The listing builds one solid part. Answer for the finished solid, in the listing's coordinates (mm). Face numbers are marked on the shaded views. Coordinates: 2 decimals unless noted, no trailing zeros. Order: outer loops, then holes, each group sorted by start corner. A loop starts at its lowest first (then second) coordinate and runs counter-clockwise, first axis right, second up. Notation, with made-up numbers: (63, 53.25) -> (116, 53.25) arc R27 ccw to (116, 91.25) -> close; hole circle Ø4 at (53, 67). An arc over 180 degrees is marked (long way). Answer in a Markdown table with one row per item. Add a question column.
```python
from build123d import *

# Parameters (mm, degrees)
SKETCH1_W           = 321.435935394
SKETCH1_H           = 221.435935394
BOSS_EXTRUDE1_DEPTH = 30
FILLET1_R           = 20
SHELL1_T            = -2
CUT_EXTRUDE1_REACH  = 1355.856
SKETCH2_W           = 156.2
SKETCH2_H           = 88.6
SKETCH5_R           = 5
SKETCH5_R_2         = 1.5
BOSS_EXTRUDE2_DEPTH = 20
FILLET2_R           = 5


with BuildPart() as part:
    # Sketch1 → Boss-Extrude1 (new body)
    with BuildSketch(Plane(origin=(0, -69.673086457, -260.023498579), x_dir=(1, 0, 0), z_dir=(0, 0.2588190451025214, 0.9659258262890682))):
        with Locations((1020.211286357, 547.548055232)):
            Rectangle(SKETCH1_W, SKETCH1_H)
    extrude(amount=BOSS_EXTRUDE1_DEPTH)

    # Fillet1
    fillet1_edges = [part.edges().sort_by_distance(p)[0] for p in [
        (859.49331866, 466.982292579, -372.761588593),
        (1020.211286357, 360.036948146, -344.105669918),
        (1180.929254054, 466.982292579, -372.761588593),
        (1020.211286357, 573.927637012, -401.417507268),
    ]]
    fillet(fillet1_edges, radius=FILLET1_R)

    # Shell1
    shell1_openings = [part.faces().sort_by_distance(p)[0] for p in [
        (1020.211286357, 459.217721226, -401.739363381),
    ]]
    offset(amount=SHELL1_T, openings=shell1_openings)

    # Sketch2 → Cut-Extrude1 (cut, up to next)
    with BuildSketch(Plane(origin=(0, -61.908515104, -231.04572379), x_dir=(1, 0, 0), z_dir=(0, 0.2588190451025213, 0.9659258262890681)), mode=Mode.PRIVATE) as cut_extrude1_sk1:
        with Locations((1020.211286357, 547.548055232)):
            Rectangle(SKETCH2_W, SKETCH2_H)
    cut_extrude1_tool1 = extrude(cut_extrude1_sk1.sketch, amount=-CUT_EXTRUDE1_REACH, mode=Mode.PRIVATE) & part.part
    add(cut_extrude1_tool1.solids().sort_by_distance((1020.211286, 466.982293, -372.761589))[0], mode=Mode.SUBTRACT)

    # Sketch5 → Boss-Extrude2 (add)
    # profile 1 of 4: a face of its own
    with BuildSketch(Plane(origin=(0, -62.426153194, -232.977575442), x_dir=(-1, 0, 0), z_dir=(0, -0.25881904510252146, -0.9659258262890681))):
        with Locations(Location((-901.394461057, 616.364880532, 0), (0, 0, 270))):
            Circle(SKETCH5_R)
        with Locations(Location((-901.394461057, 616.364880532, 0), (0, 0, 90))):
            Circle(SKETCH5_R_2, mode=Mode.SUBTRACT)
    # profile 2 of 4: a face of its own
    with BuildSketch(Plane(origin=(0, -62.426153194, -232.977575442), x_dir=(-1, 0, 0), z_dir=(0, -0.25881904510252146, -0.9659258262890681))):
        with Locations(Location((-901.394461057, 478.731229931, 0), (0, 0, 270))):
            Circle(SKETCH5_R)
        with Locations(Location((-901.394461057, 478.731229931, 0), (0, 0, 90))):
            Circle(SKETCH5_R_2, mode=Mode.SUBTRACT)
    # profile 3 of 4: a face of its own
    with BuildSketch(Plane(origin=(0, -62.426153194, -232.977575442), x_dir=(-1, 0, 0), z_dir=(0, -0.25881904510252146, -0.9659258262890681))):
        with Locations(Location((-1139.028111658, 478.731229931, 0), (0, 0, 270))):
            Circle(SKETCH5_R)
        with Locations(Location((-1139.028111658, 478.731229931, 0), (0, 0, 90))):
            Circle(SKETCH5_R_2, mode=Mode.SUBTRACT)
    # profile 4 of 4: a face of its own
    with BuildSketch(Plane(origin=(0, -62.426153194, -232.977575442), x_dir=(-1, 0, 0), z_dir=(0, -0.25881904510252146, -0.9659258262890681))):
        with Locations(Location((-1139.028111658, 616.364880532, 0), (0, 0, 270))):
            Circle(SKETCH5_R)
        with Locations(Location((-1139.028111658, 616.364880532, 0), (0, 0, 90))):
            Circle(SKETCH5_R_2, mode=Mode.SUBTRACT)
    extrude(amount=BOSS_EXTRUDE2_DEPTH)

    # Fillet2
    fillet2_edges = [part.edges().sort_by_distance(p)[0] for p in [
        (901.394461057, 537.766232461, -393.798640482),
        (901.394461057, 404.822334779, -358.17643046),
        (1139.028111658, 404.822334779, -358.17643046),
        (1139.028111658, 537.766232461, -393.798640482),
    ]]
    fillet(fillet2_edges, radius=FILLET2_R)


solid = part.part
```
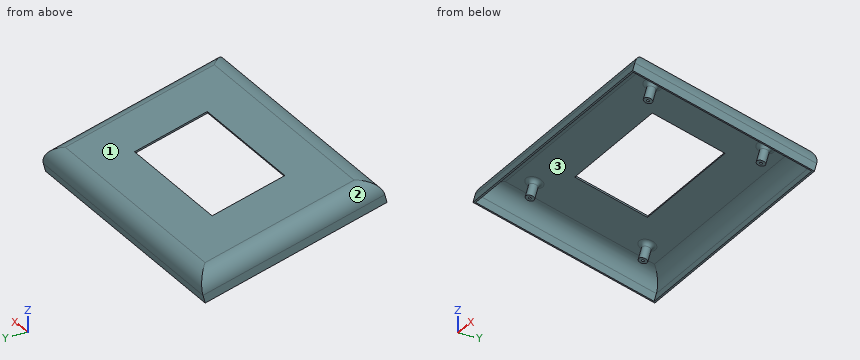
Q1. Given pin 1 (12.5 mm diameter, centred on y = 478, z = -374, fed in from -X); pin 2 (7.5 mm diameter, centred on y = 472.5, z = -379, fed in from +X); pin 3 (4 mm diameter, centred on x = 922.5, y = 427, fed in from +Z), each flat-ended and moving along its own axis, determine where each tip first touches the part or whether it passes through.
Q2. Determine the mould class of the marked faces 1, 2 and 3 for opening direction X: +X half, -X half, draft (parallel to the pull), parting line (faces both ways), or undercut.
Q3. A cutting plane is placed at A-A (x = 1018.5). Determine the outline of the cut face in (y, z), then the cut area to 3 significant figures.
Q4. A cutting plane is placed at B-B (z = -402.5). State how many separate pieces and enclosed holes the cut face has, then the cut area to 3 significant figures.
Q5. A cutting plane is placed at C-C (x = 930.5). Determine the outline of the cut face in (y, z), then the cut area to 3 significant figures.
Q6. Straight lines are drawn through the part: line 1 (X direction, y = 430, z = -384.5); line 2 (Y direction, x = 1135, z = -409); line 3 (X direction, y = 508, z = -388). For each, find the intervals that lie inside material, in ascending order.
Returned:
| question | item | result |
|---|---|---|
| 1 | pin 1 | stops at x = 866.74 |
| 1 | pin 2 | stops at x = 1177.18 |
| 1 | pin 3 | stops at z = -361.51 |
| 2 | face 1 | draft |
| 2 | face 2 | -X half |
| 2 | face 3 | undercut |
| 3 | outline | (352.27, -373.08) -> (354.2, -373.6) -> (356.79, -363.94) arc R18 cw to (378.84, -351.21) -> (423.67, -363.23) -> (424.19, -361.3) -> (379.36, -349.28) arc R20 ccw to (354.86, -363.42) -> close; (509.26, -386.16) -> (554.09, -398.17) arc R18 cw to (566.82, -420.22) -> (564.23, -429.88) -> (566.16, -430.4) -> (568.75, -420.74) arc R20 ccw to (554.61, -396.24) -> (509.77, -384.23) -> close |
| 3 | area | 345 mm² |
| 4 | separate pieces | 3 |
| 4 | enclosed holes | 2 |
| 4 | area | 1,430 mm² |
| 5 | outline | (352.27, -373.08) -> (354.2, -373.6) -> (356.79, -363.94) arc R18 cw to (378.84, -351.21) -> (554.09, -398.17) arc R18 cw to (566.82, -420.22) -> (564.23, -429.88) -> (566.16, -430.4) -> (568.75, -420.74) arc R20 ccw to (554.61, -396.24) -> (379.36, -349.28) arc R20 ccw to (354.86, -363.42) -> close |
| 5 | area | 522 mm² |
| 6 | line 1 | x = 859.49 to 861.49, 1178.93 to 1180.93 |
| 6 | line 2 | y = 525.45 to 531.58, 566.19 to 568.33 |
| 6 | line 3 | x = 867.36 to 871.05, 1169.37 to 1173.07 |
